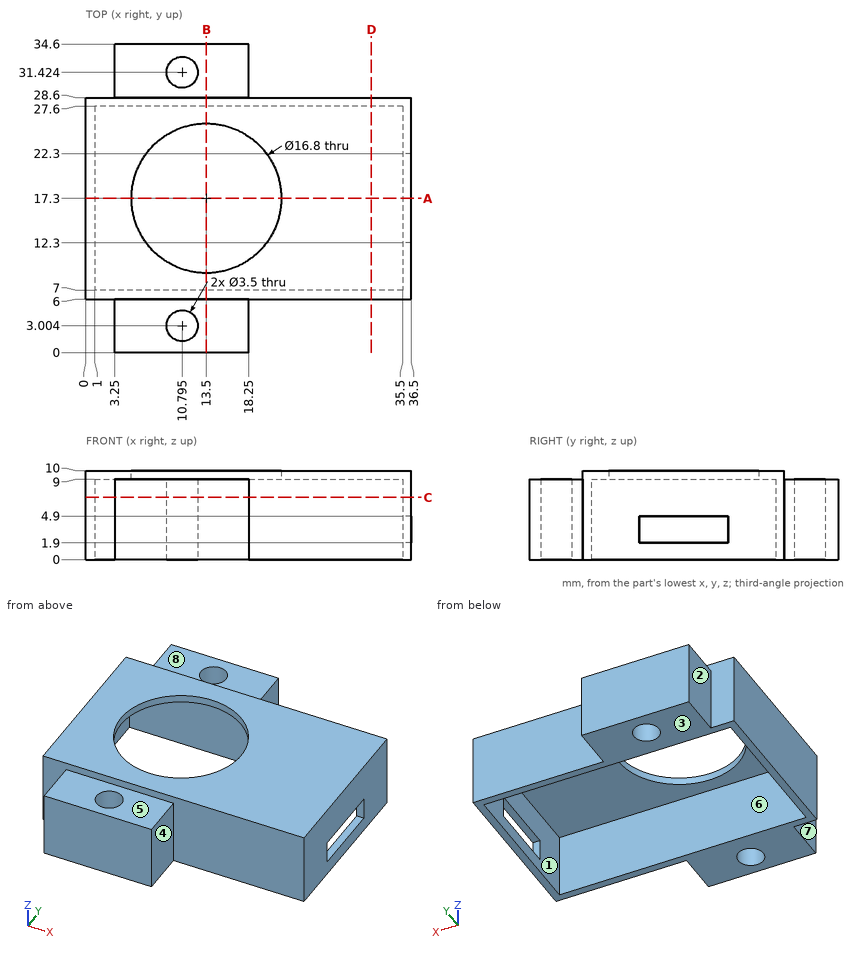
Job drawing, mm, ordinate dimensions from the low corner. One solid piece. A direction names the side the tool comes from. Round coordinates to 2 decimals unless told otherwise and drop trailing zeros. Loops run counter-clockwise (first coordinate to the right, second up) from the corner with the lowest first, then second, coordinate; pieces in that order, holes last. Notation, with made-up numbers: (-27.75, 80.5) -> (22.25, 80.5) arc R15 ccw to (22.25, 88.5) -> close; hole circle Ø6 at (80.5, 46.5). An arc over 180 degrees is marked (long way). Use CSV: the item, a comma, the result in double quotes. Start each with the question number.
Q1. Saw through at D-D on x = 32. Give the cut face in (y, z).
Q2. Saw through at C-C on z = 7. Count the separate pieces of the cut face and the enclosed holes in it, and give its area (3 significant figures).
Q3. Flat gauge pins, fed straight in: pin 1 Ø1.8 at (y, z) = (3, 5) entering from -X; pin 2 Ø5 at (x, z) = (23.5, 6.5) entering from -Y; pin 3 Ø4.5 at (y, z) = (21, 3) entering from +X; pin 4 Ø4.5 at (x, y) = (10.79, 31.42) entering from +Z. Where does each tip first touch, or does it go through?
Q4. Drill centre lines: L1, parallel to Y at x = 29, z = 7; L2, parallel to X at y = 24, z = 1.5; L3, parallel to Y at x = 13.5, z = 9.25. Where is each one in solid material? Low to high.
Q5. Which spindle directions (+Z, -Z, +X, -X, +Y, -Y) get a long thin tool onto all of the face, cutting with end or side? Do the marked faces 4, 5, 6, 7 and 8. Say none if no direction does.
Q6. Saw through at A-A on y = 17.3. Give the cut face in (x, z), and give its area (3 significant figures).
Q7. Mould opens along X. For the marked faces 1, 2 and 3 say: +X half, -X half, draft (parallel to the pull), parting line (faces both ways), or undercut.
Q8. Saw through at B-B on x = 13.5. Give the cut face in (y, z), and give its area (3 significant figures).
Solutions:
1,outline,"(6, 0) -> (7, 0) -> (7, 9) -> (27.6, 9) -> (27.6, 0) -> (28.6, 0) -> (28.6, 10) -> (6, 10) -> close"
2,separate pieces,"1"
2,enclosed holes,"3"
2,area,"275 mm^2"
3,pin 1,"stops at x = 3.25"
3,pin 2,"stops at y = 6"
3,pin 3,"stops at x = 36.5"
3,pin 4,"stops at z = 9"
4,L1,"y = 6 to 7, 27.6 to 28.6"
4,L2,"x = 0 to 1, 35.5 to 36.5"
4,L3,"y = 6 to 8.9, 25.7 to 28.6"
5,face 4,"+Z, -Z, +X, -Y"
5,face 5,"+Z, +X, -X, -Y"
5,face 6,"-Z"
5,face 7,"+Z, -Z, -X, -Y"
5,face 8,"+Z, +X, -X, +Y"
6,outline,"(0, 0) -> (1, 0) -> (1, 9) -> (5.1, 9) -> (5.1, 10) -> (0, 10) -> close; (21.9, 9) -> (35.5, 9) -> (35.5, 4.9) -> (36.5, 4.9) -> (36.5, 10) -> (21.9, 10) -> close; (35.5, 0) -> (36.5, 0) -> (36.5, 1.9) -> (35.5, 1.9) -> close"
6,area,"34.7 mm^2"
7,face 1,"undercut"
7,face 2,"-X half"
7,face 3,"draft"
8,outline,"(0, 0) -> (7, 0) -> (7, 9) -> (8.9, 9) -> (8.9, 10) -> (6, 10) -> (6, 9) -> (0, 9) -> close; (25.7, 9) -> (27.6, 9) -> (27.6, 0) -> (34.6, 0) -> (34.6, 9) -> (28.6, 9) -> (28.6, 10) -> (25.7, 10) -> close"
8,area,"132 mm^2"
